Build history of the part. All positions in model axes, mm. A direction names the side the tool comes from. Give positions to 0.01 mm unless a question says otherwise; leave off trailing zeros. Order: outer loops, then holes, each group sorted by start corner. A loop starts at its lowest first (then second) coordinate and runs counter-clockwise, first axis right, second up. Notation, with made-up numbers: (-27.5, 67) - (20.5, 67) arc R7 ccw to (20.5, 77) - close; hole circle Ø9 at (-30, -37). An arc over 180 degrees is marked (long way). Use a Markdown table: item, result.
from build123d import *

# Parameters (mm, degrees)
BOSS_EXTRUDE1_DEPTH                                 = 7.5
CBORE_FOR_M4_HEX_SOCKET_HEAD_CAP_SCREW2_D           = 4.8
CBORE_FOR_M4_HEX_SOCKET_HEAD_CAP_SCREW2_CBORE_D     = 8
CBORE_FOR_M4_HEX_SOCKET_HEAD_CAP_SCREW2_CBORE_DEPTH = 4.4
CHAMFER1_SIZE                                       = 30
CHAMFER1_SIZE_2                                     = 15
FILLET1_R                                           = 1
CHAMFER2_SIZE                                       = 1


# Some blends are built 0.0001 mm under size
with BuildPart() as part:
    # Sketch2 → Boss-Extrude1 (new, symmetric)
    with BuildSketch(Plane(origin=(0, 0, 0), x_dir=(1, 0, 0), z_dir=(0, 1, 0))):
        Polygon((0, 0), (0, 70), (-57.8, 70), (-57.8, 60), (-27.8, 60), (-27.8, 55.1), (-10, 55.1), (-10, 34.9), (-27.8, 34.9), (-27.8, 0), align=None)
    extrude(amount=BOSS_EXTRUDE1_DEPTH, both=True)

    # Sketch4 → CBORE for M4 Hex Socket Head Cap Screw1 (revolve, cut)
    with BuildSketch(Plane(origin=(0, 0, -15), x_dir=(0, 0, -1), z_dir=(0, 1, 0))):
        Polygon((0, 0), (0, 27.8), (2.4, 27.8), (2.4, 22), (4, 22), (4, 0.025), (4.025, 0), align=None)
    revolve(axis=Axis((6.35, 0, -15), (-1, 0, 0)), mode=Mode.SUBTRACT)

    # CBORE for M4 Hex Socket Head Cap Screw2 (through all)
    with Locations(Plane(origin=(0, 0, -70), x_dir=(-1, 0, 0), z_dir=(0, 0, -1))):
        with Locations((42.8, 0)):
            CounterBoreHole(CBORE_FOR_M4_HEX_SOCKET_HEAD_CAP_SCREW2_D / 2, CBORE_FOR_M4_HEX_SOCKET_HEAD_CAP_SCREW2_CBORE_D / 2, CBORE_FOR_M4_HEX_SOCKET_HEAD_CAP_SCREW2_CBORE_DEPTH)

    # Chamfer1
    # the kernel refuses this chamfer: 30, 15 mm, written as the material it takes off along each edge
    with BuildSketch(Plane(origin=(0, 85.194866214, 0), x_dir=(0.01726807512366813, 0, -0.9998508956747117), z_dir=(0, -1, 0))) as chamfer1_piece_1:
        Polygon((CHAMFER1_SIZE * 0.999850895675, -CHAMFER1_SIZE * 0.0172680751237), (-CHAMFER1_SIZE_2 * 0.0172680751237, -CHAMFER1_SIZE_2 * 0.999850895675), (0, 0), align=None)
    extrude(amount=170.389732427, mode=Mode.SUBTRACT)

    # Fillet1
    fillet1_edges = [part.edges().sort_by_distance(p)[0] for p in [
        (0, 0, -70),
        (-27.8, 0, 0),
        (-27.8, 0, -34.9),
        (-10, 0, -34.9),
        (-10, 0, -55.1),
        (-27.8, 0, -55.1),
        (-27.8, 0, -60),
        (-57.8, 0, -60),
        (-57.8, 0, -70),
        (0, 0, -30),
        (-15, 0, 0),
    ]]
    fillet(fillet1_edges, radius=FILLET1_R)

    # Chamfer2
    chamfer2_edges = [part.edges().sort_by_distance(p)[0] for p in [
        (-28.092893219, -7.5, -59.707106781),
        (-28.092893219, 7.5, -59.707106781),
        (-10.292893219, -7.5, -35.192893219),
        (-10.292893219, 7.5, -35.192893219),
        (-10.292893219, -7.5, -54.807106781),
        (-10.292893219, 7.5, -54.807106781),
        (-27.8, -7.5, -57.55),
        (-27.8, 7.5, -57.55),
        (-42.8, -7.5, -60),
        (-42.8, 7.5, -60),
        (-18.9, -7.5, -34.9),
        (-18.9, 7.5, -34.9),
        (-10, -7.5, -45),
        (-10, 7.5, -45),
        (-18.9, -7.5, -55.1),
        (-18.9, 7.5, -55.1),
        (-57.8, -7.5, -65),
        (-57.8, 7.5, -65),
        (0, -7.5, -49.618033989),
        (-7.414589803, -7.5, -15.170820393),
        (-21.209016994, -7.5, 0),
        (-27.8, -7.5, -17.45),
        (-28.9, -7.5, -70),
        (-27.507106781, -7.5, -55.392893219),
        (-27.507106781, -7.5, -34.607106781),
        (-57.507106781, -7.5, -60.292893219),
        (-27.507106781, -7.5, -0.292893219),
        (-15.092302877, -7.5, -0.149349192),
        (-0.026751011, -7.5, -30.006315057),
        (-0.292893219, -7.5, -69.707106781),
        (-57.507106781, -7.5, -69.707106781),
        (-28.9, 7.5, -70),
        (-21.209016994, 7.5, 0),
        (-7.414589803, 7.5, -15.170820393),
        (0, 7.5, -49.618033989),
        (-27.8, 7.5, -17.45),
        (-27.507106781, 7.5, -55.392893219),
        (-27.507106781, 7.5, -34.607106781),
        (-57.507106781, 7.5, -60.292893219),
        (-27.507106781, 7.5, -0.292893219),
        (-15.092302877, 7.5, -0.149349192),
        (-0.026751011, 7.5, -30.006315057),
        (-0.292893219, 7.5, -69.707106781),
        (-57.507106781, 7.5, -69.707106781),
    ]]
    chamfer(chamfer2_edges, length=CHAMFER2_SIZE - 0.0001)  # a hair under: the kernel refuses the full size


solid = part.part
1) Pin check, flat tips, straight feed: P1, Ø6, axis at y = 0, z = -15, coming from the -X side; P2, Ø6.5, axis at x = -42.8, y = 0, coming from the -Z side; P3, Ø2, axis at x = -27, z = -12, coming from the -Y side; P4, Ø9, axis at y = 0.5, z = -15, coming from the +X side. Stop position of each tip, or through.
Computed:
| item | result |
|---|---|
| P1 | stops at x = -27.8 |
| P2 | stops at z = -65.6 |
| P3 | stops at y = -7.5 |
| P4 | stops at x = -5.25 |
2) Tool access for faces 4 (the flat face through (-19, 0, -34.9)), 5 (the flat face through (-22, 2, -13)), 6 (the conical face through (-10.034, 6.882, -34.912)), 7 (the cylindrical face through (-46.615, 1.201, -67.831)): list every direction of +Z, -Z, +X, -X, +Y, -Y with a clear straight run to the whole face (end or side of a thin tool).
Computed:
| item | result |
|---|---|
| face 4 | -X, +Y, -Y |
| face 5 | +X |
| face 6 | -X, +Y |
| face 7 | -Z |
3) Two-plate mould, pull along Z, no slides. Class faces 1 (the flat face through (-29, 0, -70)), 2 (the conical face through (-10.034, -6.882, -34.912)), 3 (the flat face through (-7.75, -6.99, -15.6)): +Z half, -Z half, draft (parallel to the pull), parting line (faces both ways), or undercut.
Computed:
| item | result |
|---|---|
| face 1 | -Z half |
| face 2 | undercut |
| face 3 | +Z half |
4) Slice it at A-A (x = -12). Write the cut outline in (y, z), and give its area (4 significant figures).
Computed:
| item | result |
|---|---|
| outline | (-7.5, -69) - (-6.5, -70) - (6.5, -70) - (7.5, -69) - (7.5, -56.1) - (6.5, -55.1) - (-6.5, -55.1) - (-7.5, -56.1) - close; (-7.5, -33.9) - (-6.5, -34.9) - (6.5, -34.9) - (7.5, -33.9) - (7.5, -8.24) - (6.5, -6) - (-6.5, -6) - (-7.5, -8.24) - close; hole circle Ø8 at (0, -15) |
| area | 601.5 mm² |
5) Slice it at B-B (x = -42.8). Write the cut outline in (y, z), and give its area (3 significant figures).
Computed:
| item | result |
|---|---|
| outline | (-7.5, -69) - (-6.5, -70) - (-4, -70) - (-4, -65.6) - (-2.4, -65.6) - (-2.4, -60) - (-6.5, -60) - (-7.5, -61) - close; (2.4, -65.6) - (4, -65.6) - (4, -70) - (6.5, -70) - (7.5, -69) - (7.5, -61) - (6.5, -60) - (2.4, -60) - close |
| area | 85.9 mm² |
6) Slice it at D-D (z = -15). Write the cut outline in (x, y).
Computed:
| item | result |
|---|---|
| outline | (-27.8, -6.5) - (-26.8, -7.5) - (-8.62, -7.5) - (-7.5, -6.5) - (-7.5, -4) - (-22, -4) - (-22, -2.4) - (-27.8, -2.4) - close; (-27.8, 2.4) - (-22, 2.4) - (-22, 4) - (-7.5, 4) - (-7.5, 6.5) - (-8.62, 7.5) - (-26.8, 7.5) - (-27.8, 6.5) - close |
7) Slice it at C-C (z = -39.5). Write the cut outline in (x, y), and give its area (3 significant figures).
Computed:
| item | result |
|---|---|
| outline | (-10, -6.5) - (-9, -7.5) - (-1, -7.5) - (0, -6.5) - (0, 6.5) - (-1, 7.5) - (-9, 7.5) - (-10, 6.5) - close |
| area | 148 mm² |
8) Wall check: line 1 (Z direction, x = -24.75, y = 0); line 2 (Z direction, x = -16.25, y = 0); line 3 (Y direction, x = -42.8, z = -68.65). Give the ranges that are in metal, low to high. Write a range as from..to.
Computed:
| item | result |
|---|---|
| line 1 | z = -70..-55.1, -34.9..-17.4, -12.6..0 |
| line 2 | z = -70..-55.1, -34.9..-19, -11..0 |
| line 3 | y = -7.5..-4, 4..7.5 |
